Geometry check sheet. Reference: the model listing, model coordinates, mm. A direction names the side the tool comes from. Give positions to 0.01 mm unless a question says otherwise; leave off trailing zeros. Order: outer loops, then holes, each group sorted by start corner. A loop starts at its lowest first (then second) coordinate and runs counter-clockwise, first axis right, second up. Notation, with made-up numbers: M 59,23.5 L 85,23.5 A25 ccw 85,54.5 Z; hole C -21,-13 d7. An arc over 180 degrees is marked long. Put each result on its own line as item: value. Start each with the question number.
Q1. Section check A-A on y = -14.5. Record the cut outline in (x, z).
Q2. Section check B-B on z = 29. Record the cut outline in (x, y).
Q3. Go/stop test with flat-tipped pins: pin 1 (2.5 mm diameter, centred on y = -41, z = 16.5, fed in from +X); pin 2 (4 mm diameter, centred on y = -22, z = 26.5, fed in from +X); pin 3 (4 mm diameter, centred on y = 16.5, z = 37.5, fed in from +X). Record where each tip stops, or that it passes through.
Q4. Mould release check, pull along Y, two halves, no side actions. Record for faces 1 (the flat face through (-4, -1, 47)), 2 (the flat face through (-11, -42.995, 17)), 3 (the cylindrical face through (-64.846, 17.43, 1.479)): +Y half, -Y half, draft (parallel to the pull), parting line (faces both ways), or undercut.
Q5. Access from +Z, -Z, +X, -X, +Y, -Y to the whole of each face (thin tool, end or side, straight path). Record for faces 4 (the flat face through (-6, 38, 23)), 5 (the flat face through (-4, 36.005, 11)), 6 (the flat face through (36.04, -41, 13)), 7 (the flat face through (42.04, -18, 2)), 8 (the flat face through (39.04, 16, 27)).
Q6. Material ranges on L1, parallel to Y at x = -38.5, z = 22.5; L2, parallel to X at y = 17.5, z = 46.5; L3, parallel to X at y = -4, z = 25.5, recorded low to high.
Q7. Section check C-C on x = -44. Record the cut outline in (y, z), then the cut area to 3 significant figures.
Q8. Section check D-D on z = 20. Record the cut outline in (x, y).
```python
from build123d import *

# Parameters (mm, degrees)
SKETCH_1_W          = 147
SKETCH_1_H          = 82
EXTRUDE_1_DEPTH     = 50
SKETCH_2_W          = 29.5
SKETCH_2_H          = 82
CUT_EXTRUDE_1_DEPTH = 47
SKETCH_3_W          = 29.5
SKETCH_3_H          = 82
CUT_EXTRUDE_2_DEPTH = 47
SKETCH_5_W          = 82
SKETCH_5_H          = 76
CUT_EXTRUDE_3_DEPTH = 47
SKETCH_6_R          = 2.4
CUT_EXTRUDE_4_DEPTH = 4
SKETCH_7_W          = 82
SKETCH_7_H          = 24
CUT_EXTRUDE_5_DEPTH = 84
SKETCH_9_W          = 44
SKETCH_9_H          = 47
CUT_EXTRUDE_6_DEPTH = 3
SKETCH_10_W         = 6
SKETCH_10_H         = 44
CUT_EXTRUDE_7_DEPTH = 7
SKETCH_12_R         = 1.5
CUT_EXTRUDE_8_DEPTH = 3


with BuildPart() as part:
    # 草图1 → 凸台-拉伸1 (new body)
    with BuildSketch(Plane.XY):
        with Locations((-4.960122699, -1.995398773)):
            Rectangle(SKETCH_1_W, SKETCH_1_H)
    extrude(amount=EXTRUDE_1_DEPTH)

    # 草图2 → 切除-拉伸1 (cut)
    with BuildSketch(Plane.XY.offset(50)):
        with Locations((-63.710122699, -1.995398773)):
            Rectangle(SKETCH_2_W, SKETCH_2_H)
    extrude(amount=-CUT_EXTRUDE_1_DEPTH, mode=Mode.SUBTRACT)

    # 草图3 → 切除-拉伸2 (cut)
    with BuildSketch(Plane.XY.offset(50)):
        with Locations((53.789877301, -1.995398773)):
            Rectangle(SKETCH_3_W, SKETCH_3_H)
    extrude(amount=-CUT_EXTRUDE_2_DEPTH, mode=Mode.SUBTRACT)

    # 草图5 → 切除-拉伸3 (cut)
    with BuildSketch(Plane(origin=(0, 0, 0), x_dir=(-1, 0, 0), z_dir=(0, 0, -1))):
        with Locations((4.960122699, -1.995398773)):
            Rectangle(SKETCH_5_W, SKETCH_5_H)
    extrude(amount=-CUT_EXTRUDE_3_DEPTH, mode=Mode.SUBTRACT)

    # 草图6 → 切除-拉伸4 (cut)
    with BuildSketch(Plane.XY.offset(50)):
        with Locations((-4.960122699, 24.004601227)):
            Circle(SKETCH_6_R)
    extrude(amount=-CUT_EXTRUDE_4_DEPTH, mode=Mode.SUBTRACT)

    # 草图7 → 切除-拉伸5 (cut)
    with BuildSketch(Plane(origin=(0, 39.004601227, 0), x_dir=(1, 0, 0), z_dir=(0, 1, 0))):
        with Locations((-4.960122699, -35)):
            Rectangle(SKETCH_7_W, SKETCH_7_H)
    extrude(amount=-CUT_EXTRUDE_5_DEPTH, mode=Mode.SUBTRACT)

    # 草图9 → 切除-拉伸6 (cut)
    with BuildSketch(Plane(origin=(39.039877301, 0, 0), x_dir=(0, 0, -1), z_dir=(1, 0, 0))):
        with Locations((-25, -19.495398773)):
            Rectangle(SKETCH_9_W, SKETCH_9_H)
    extrude(amount=-CUT_EXTRUDE_6_DEPTH, mode=Mode.SUBTRACT)

    # 草图10 → 切除-拉伸7 (cut)
    with BuildSketch(Plane.XY.offset(3)):
        with Locations((39.039877301, -17.995398773)):
            Rectangle(SKETCH_10_W, SKETCH_10_H)
    extrude(amount=-CUT_EXTRUDE_7_DEPTH, mode=Mode.SUBTRACT)

    # 草图12 → 切除-拉伸8 (cut)
    with BuildSketch(Plane(origin=(0, 0, 0), x_dir=(-1, 0, 0), z_dir=(0, 0, -1))):
        with Locations((63.460122699, 18.004601227)):
            Circle(SKETCH_12_R)
        with Locations((63.460122699, -21.995398773)):
            Circle(SKETCH_12_R)
        with Locations((-53.539877301, 18.004601227)):
            Circle(SKETCH_12_R)
        with Locations((-53.539877301, -21.995398773)):
            Circle(SKETCH_12_R)
    extrude(amount=-CUT_EXTRUDE_8_DEPTH, mode=Mode.SUBTRACT)


solid = part.part
```
Results found:
1. outline: M -78.46,0 L -45.96,0 L -45.96,47 L 39.04,47 L 39.04,50 L -48.96,50 L -48.96,3 L -78.46,3 Z; M 42.04,0 L 68.54,0 L 68.54,3 L 42.04,3 Z
2. outline: M -48.96,-43 L -45.96,-43 L -45.96,39 L -48.96,39 Z; M 36.04,4 L 39.04,4 L 39.04,39 L 36.04,39 Z
3. pin 1: stops at x = 36.04
3. pin 2: stops at x = -45.96
3. pin 3: stops at x = 39.04
4. face 1: draft
4. face 2: -Y half
4. face 3: undercut
5. face 4: +Y, -Y
5. face 5: -Z
5. face 6: +X, -Y
5. face 7: +Z, -Z
5. face 8: +Z, +X, +Y, -Y
6. L1: y = -43 to -40, 36 to 39
6. L2: x = -48.96 to -45.96, 36.04 to 39.04
6. L3: x = -48.96 to -45.96
7. outline: M -43,0 L -40,0 L -40,23 L -43,23 Z; M -43,47 L 39,47 L 39,50 L -43,50 Z; M 36,0 L 39,0 L 39,23 L 36,23 Z
7. area: 384 mm^2
8. outline: M -48.96,-43 L 36.04,-43 L 36.04,-40 L -45.96,-40 L -45.96,36 L 36.04,36 L 36.04,4 L 39.04,4 L 39.04,39 L -48.96,39 Z
